```python
from build123d import *

# Parameters (mm, degrees)
F1_DEPTH = 0.6
F2_W     = 4.5
F2_H     = 2.2
F3_DEPTH = 1.6
F4_R     = 1.09999
F5_R     = 0.5
F6_DEPTH = 25


# Not quite as in the source:
# - a fillet or chamfer is up to 0.001 mm smaller than in the source, because OpenCascade refuses the exact size


with BuildPart() as f1:
    # F0 (on Top) → F1 (new body)
    with BuildSketch(Plane.XY):
        with BuildLine():
            Line((11.0937791562, 2.9), (15.5, 2.9))
            Line((15.5, 2.9), (15.5, 5.1))
            Line((15.5, 5.1), (11.0937791562, 5.1))
            ThreePointArc((11.0937791562, 5.1), (10.0387329979, 5.2416483307), (9.0584096032, 5.656561198))
            Line((9.0584096032, 5.656561198), (6.035369553, 7.443438802))
            ThreePointArc((6.035369553, 7.443438802), (5.0550461583, 7.8583516693), (4, 8))
            Line((4, 8), (4, 6.65))
            ThreePointArc((4, 6.65), (5.8738329701, 5.8738329701), (6.65, 4))
            ThreePointArc((6.65, 4), (5.8738329701, 2.1261670299), (4, 1.35))
            Line((4, 1.35), (4, 0))
            ThreePointArc((4, 0), (5.0550461583, 0.1416483307), (6.035369553, 0.556561198))
            Line((6.035369553, 0.556561198), (9.0584096032, 2.343438802))
            ThreePointArc((9.0584096032, 2.343438802), (10.0387329979, 2.7583516693), (11.0937791562, 2.9))
        make_face()
        with BuildLine():
            ThreePointArc((0, 4), (1.1715728753, 1.1715728753), (4, 0))
            Line((4, 0), (4, 1.35))
            ThreePointArc((4, 1.35), (1.35, 4), (4, 6.65))
            Line((4, 6.65), (4, 8))
            ThreePointArc((4, 8), (1.1715728753, 6.8284271247), (0, 4))
        make_face()
    extrude(amount=F1_DEPTH)

    # F2 (on face) → F3 (join)
    with BuildSketch(Plane.XY.offset(0.6)):
        with Locations((13.25, 4)):
            Rectangle(F2_W, F2_H)
    extrude(amount=F3_DEPTH)

    # F4 (radius 1.1 in the source; OpenCascade refuses exactly that, so slightly less here)
    f4_edges = [f1.edges().sort_by_distance(p)[0] for p in [
        (13.25, 5.1, 2.2),
        (13.25, 2.9, 2.2),
    ]]
    fillet(f4_edges, radius=F4_R)

    # F5 (on face) → F6 (cut)
    with BuildSketch(Plane.YZ.offset(15.5)):
        with Locations((4, 1.1)):
            Circle(F5_R)
    extrude(amount=-F6_DEPTH, mode=Mode.SUBTRACT)


solid = f1.part
```
Check sheet for the modelled part. Datum: model origin and axes. Units: mm. A direction names the side the tool comes from. Give positions to 0.01 mm unless a question says otherwise; leave off trailing zeros. Write each loop counter-clockwise with the first axis right and the second up, starting at its lowest first coordinate (ties: lowest second). Pieces come first, ordered by that corner, then holes.
Item 1: Cross-section at D-D (y = 1). Enter the section's corners in (x, z).
Item 2: Draft check along Y on faces 4 (the face through (13.282, 3.231, 1.886)), 5 (the face through (8, 4, 0)), 6 (the face through (13.3, 3.6, 1.4)), 7 (the face through (7.568, 6.537, 0.296)). Enter one of: released by +Y, released by -Y, zero draft, split by the parting line, or undercut.
Item 3: Cross-section at C-C (x = 6.25). Enter the section's corners in (y, z), and give its area (3 significant figures).
Item 4: Gauge pin test, flat ends, axial feed: pin 1 (3 mm diameter, centred on x = 9.5, y = 1.5, fed in from +Z); pin 2 (1.3 mm diameter, centred on y = 3.5, z = 2, fed in from -X); pin 3 (1.2 mm diameter, centred on x = 14.5, z = 0.5, fed in from +Y). Record the tip position at first contact, or that the pin passes through.
Item 5: Cross-section at A-A (y = 2). Enter the section's corners in (x, z), and give its area (3 significant figures).
Item 6: Access from +Z, -Z, +X, -X, +Y, -Y to the whole of each face (thin tool, end or side, straight path). Record for faces 1 (the face through (13.2, 5.1, 0.5)), 2 (the face through (13.2, 2.9, 0.5)), 3 (the face through (11, 4, 2)).
Item 7: Scan lines: L1, parallel to Y at x = 12, z = 1.1; L2, parallel to Z at x = 13.55, y = 4; L3, parallel to X at y = 4.5, z = 1.45. Record each from-to range of solid material in increasing order.
Report:
1. outline: (1.35, 0) - (6.79, 0) - (6.79, 0.6) - (1.35, 0.6) - close
2. face 4: released by -Y
2. face 5: zero draft
2. face 6: undercut
2. face 7: released by +Y
3. outline: (0.68, 0) - (2.6, 0) - (2.6, 0.6) - (0.68, 0.6) - close; (5.4, 0) - (7.32, 0) - (7.32, 0.6) - (5.4, 0.6) - close
3. area: 2.30 mm2
4. pin 1: stops at z = 0.6
4. pin 2: stops at x = 11
4. pin 3: stops at y = 5.1
5. outline: (0.54, 0) - (2.26, 0) - (2.26, 0.6) - (0.54, 0.6) - close; (5.74, 0) - (8.48, 0) - (8.48, 0.6) - (5.74, 0.6) - close
5. area: 2.68 mm2
6. face 1: +Z, -Z, +X, +Y
6. face 2: +Z, -Z, +X, -Y
6. face 3: +Z, -X, +Y, -Y
7. L1: y = 2.9 to 3.5, 4.5 to 5.1
7. L2: z = 0 to 0.6, 1.6 to 2.2
7. L3: x = 11 to 15.5
